Geometry check sheet. Reference: drawing and pictorial views, mm from the part's lowest x, y, z. A direction names the side the tool comes from. Round coordinates to 2 decimals unless told otherwise and drop trailing zeros. Order: outer loops, then holes, each group sorted by start corner. A loop starts at its lowest first (then second) coordinate and runs counter-clockwise, first axis right, second up.
(1) Set-up check for the marked faces 5, 6 and 7: record each of +Z, -Z, +X, -X, +Y, -Y from which the full face is reachable in a straight line by a thin tool's end or side.
(2) Cross-section at B-B on z = 1.5. Enter the section's corners in (x, y), and give its area (3 significant figures).
(3) Cross-section at A-A on y = 15. Count the separate pieces of the cut face and the enclosed holes in it, and give its area (3 significant figures).
(4) Draft check along Y on the marked faces 1, 2, 3 and 4. Enter one of: pulls with the +Y half, pulls with the -Y half, needs draft (parallel to the pull), parting line crosses it, or undercut.
(5) Cross-section at D-D on z = 8. Enter the section's corners in (x, y) (1 decimal).
(6) Thickness scan on L1, parallel to X at y = 13.75, z = 3.75; L2, parallel to Y at x = 42, z = 3; L3, parallel to Z at x = 31, y = 6.5. Record the ranges inside material, lowest first.
(7) Gauge pin test, flat ends, axial feed: P1, Ø3, axis at x = 29.5, y = 16.5, coming from the -Z side; P2, Ø1.5, axis at y = 7.5, z = 6, coming from the -X side; P3, Ø5, axis at x = 44, z = 6, coming from the -Y side; P4, Ø3, axis at x = 19.5, z = 5, coming from the +Y side. Record the tip position at first contact, or that the pin passes through.
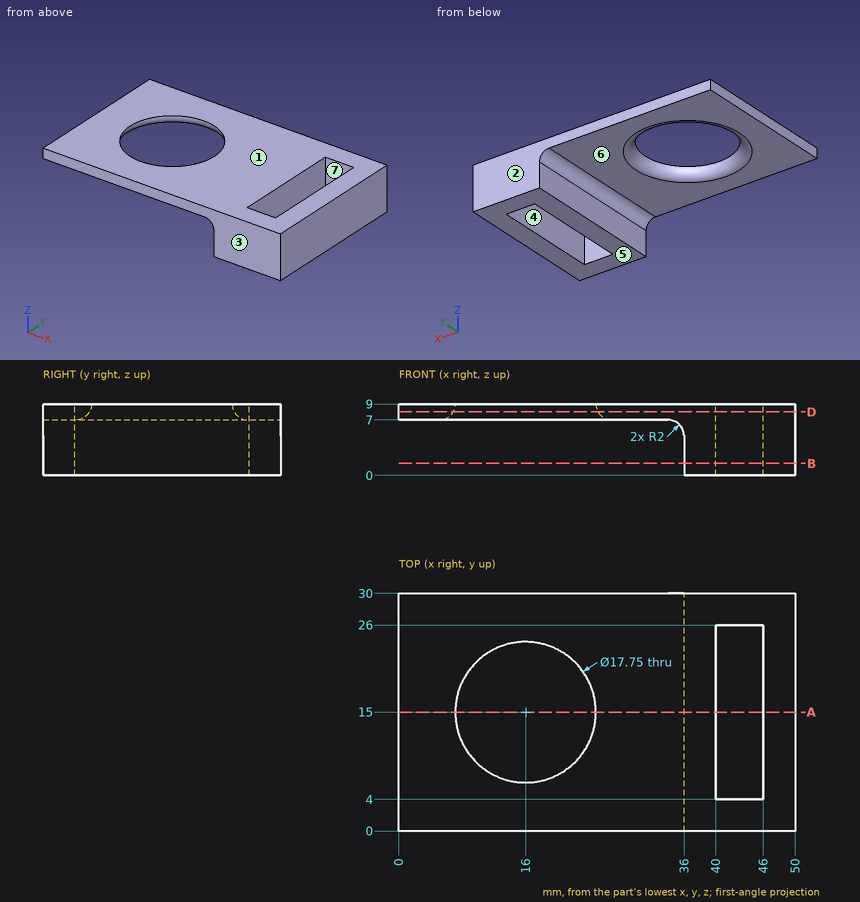
Found:
1. face 5: -Z, +X, -X, +Y, -Y
1. face 6: -Z, -X, +Y, -Y
1. face 7: +Z, -Z
2. outline: (36, 0) - (50, 0) - (50, 30) - (36, 30) - close; hole (40, 4) - (46, 4) - (46, 26) - (40, 26) - close
2. area: 288 mm2
3. separate pieces: 3
3. enclosed holes: 0
3. area: 108 mm2
4. face 1: needs draft
4. face 2: pulls with the +Y half
4. face 3: pulls with the -Y half
4. face 4: undercut
5. outline: (0, 0) - (50, 0) - (50, 30) - (0, 30) - close; hole circle Ø18.3 at (16, 15); hole (40, 4) - (46, 4) - (46, 26) - (40, 26) - close
6. L1: x = 36 to 40, 46 to 50
6. L2: y = 0 to 4, 26 to 30
6. L3: z = 7 to 9
7. P1: stops at z = 7
7. P2: stops at x = 34.97
7. P3: stops at y = 0
7. P4: passes through
